Could you check a few things on this model? Use its own coordinates, in mm. A direction names the side the tool comes from. Round coordinates to 2 decimals unless told otherwise and drop trailing zeros. Order: outer loops, then holes, each group sorted by start corner. A loop starts at its lowest first (then second) coordinate and runs counter-clockwise, first axis right, second up. Notation, with made-up numbers: (22.5, 79.25) - (75.5, 79.25) arc R31 cw to (75.5, 105.25) - close; hole circle Ø6 at (-40, 71). An arc over 180 degrees is marked (long way). Use one line per item in the form item = value.
from build123d import *

# Parameters (mm, degrees)
EXTRUDE_1_DEPTH     = 1.5
SKETCH_3_R          = 2.9
EXTRUDE_2_DEPTH     = 3.829
EXTRUDE_START       = 0.5
SKETCH_4_R          = 2.9
EXTRUDE_3_DEPTH     = 0.5
SKETCH_5_R          = 2
CUT_EXTRUDE_1_DEPTH = 3
CUT_EXTRUDE_START   = -0.7
SKETCH_6_R          = 2
CUT_EXTRUDE_2_DEPTH = 0.7
SKETCH_7_R          = 1.1
CUT_EXTRUDE_3_DEPTH = 3.7
SKETCH_8_R          = 0.75
CUT_EXTRUDE_4_DEPTH = 3.7


with BuildPart() as part:
    # 草图1 → 凸台-拉伸1 (new body)
    with BuildSketch(Plane.XY):
        with BuildLine():
            Line((-2.15, 0), (-2.797439847, -4.825584994))
            ThreePointArc((-2.797439847, -4.825584994), (0, -8.49), (2.797439847, -4.825584994))
            Line((2.797439847, -4.825584994), (2.15, 0))
            ThreePointArc((2.15, 0), (0, 2.15), (-2.15, 0))
        make_face()
    extrude(amount=EXTRUDE_1_DEPTH)

    # 草图3 → 凸台-拉伸2 (add)
    with BuildSketch(Plane.XY.offset(1.5)):
        with Locations(Location((0, -5.59, 0), (0, 0, 164.716730752))):
            Circle(SKETCH_3_R)
    extrude(amount=EXTRUDE_2_DEPTH)

    # 草图4 → 凸台-拉伸3 (add)
    with BuildSketch(Plane(origin=(0, 0, 0), x_dir=(-1, 0, 0), z_dir=(0, 0, -1)).offset(EXTRUDE_START)):
        with Locations((0, -5.59)):
            Circle(SKETCH_4_R)
    extrude(amount=-EXTRUDE_3_DEPTH)

    # 草图5 → 切除-拉伸1 (cut)
    with BuildSketch(Plane.XY.offset(5.329)):
        with Locations((0, -5.59)):
            Circle(SKETCH_5_R)
    extrude(amount=-CUT_EXTRUDE_1_DEPTH, mode=Mode.SUBTRACT)

    # 草图6 → 切除-拉伸2 (cut)
    with BuildSketch(Plane(origin=(0, 0, -0.5), x_dir=(-1, 0, 0), z_dir=(0, 0, -1)).offset(CUT_EXTRUDE_START)):
        with Locations(Location((0, -5.59, 0), (0, 0, 180))):
            Circle(SKETCH_6_R)
    extrude(amount=CUT_EXTRUDE_2_DEPTH, mode=Mode.SUBTRACT)

    # 草图7 → 切除-拉伸3 (cut)
    with BuildSketch(Plane(origin=(0, 0, 0.2), x_dir=(-1, 0, 0), z_dir=(0, 0, -1))):
        with Locations((0, -5.59)):
            Circle(SKETCH_7_R)
    extrude(amount=-CUT_EXTRUDE_3_DEPTH, mode=Mode.SUBTRACT)

    # 草图8 → 切除-拉伸4 (cut)
    with BuildSketch(Plane.XY.offset(1.5)):
        Circle(SKETCH_8_R)
    extrude(amount=-CUT_EXTRUDE_4_DEPTH, mode=Mode.SUBTRACT)


solid = part.part
Item 1: For faces 5 (the face through (0.9, -4.7, 0.2)), 6 (the face through (-2.47, -2.38, 0.74)), 7 (the face through (-0.434, -7.542, 3.85)), which set-ups out of +Z, -Z, +X, -X, +Y, -Y let a thin tool reach every point of the face, with its end or its side?
Found:
face_5 = -Z
face_6 = +Z, -Z, -X, +Y
face_7 = +Z
Item 2: Imagine slicing it at A-A on y = -5.59. Please give me the cut outline in (x, z), plus the area to 3 significant figures.
Found:
outline = (-2.9, -0.5) - (-2, -0.5) - (-2, 0.2) - (-1.1, 0.2) - (-1.1, 2.33) - (-2, 2.33) - (-2, 5.33) - (-2.9, 5.33) - close; (1.1, 0.2) - (2, 0.2) - (2, -0.5) - (2.9, -0.5) - (2.9, 5.33) - (2, 5.33) - (2, 2.33) - (1.1, 2.33) - close
area = 14.3 mm2
Item 3: I need wall thicknesses on L1, parallel to Y at x = 0, z = 0.35; L2, parallel to Y at x = 0, z = -0.1; L3, parallel to Y at x = 0.3, z = 0.35. Which ranges of each line are inside material? Lowest first, please.
Found:
L1 = -8.49 to -6.69, -4.49 to -0.75, 0.75 to 2.15
L2 = -8.49 to -7.59, -3.59 to -2.69
L3 = -8.47 to -6.65, -4.53 to -0.69, 0.69 to 2.13
Item 4: Imagine slicing it at D-D on y = -3.25. Please give me the cut outline in (x, z), plus the area to 3 significant figures.
Found:
outline = (-2.59, 0) - (-1.71, 0) - (-1.71, -0.5) - (1.71, -0.5) - (1.71, 0) - (2.59, 0) - (2.59, 1.5) - (1.71, 1.5) - (1.71, 5.33) - (-1.71, 5.33) - (-1.71, 1.5) - (-2.59, 1.5) - close
area = 22.6 mm2
Item 5: If we mould it in two halves opening along Y, with no side actions, what happens to faces 1 (the face through (0.9, -6.5, 2.329)), 2 (the face through (-0.26, -7.573, -0.145)), 3 (the face through (0.05, 2.15, 0.74)), 4 (the face through (0, -1, 1.5))? For each: released by +Y, released by -Y, zero draft, split by the parting line, or undercut.
Found:
face_1 = undercut
face_2 = undercut
face_3 = released by +Y
face_4 = zero draft
Item 6: Will these pins go through, and if not, where does the flat tip stop? P1, Ø1.5, axis at x = -1.5, z = 0.5, coming from the +Y side; P2, Ø3, axis at x = 0, y = -5.59, coming from the +Z side; P3, Ø2, axis at y = -4, z = 1.5, coming from the +X side.
Found:
P1 = 2.01
P2 = 2.33
P3 = 2.84
Item 7: Imagine slicing it at B-B on x = 0. Please give me the cut outline in (y, z), plus the area to 3 significant figures.
Found:
outline = (-8.49, -0.5) - (-7.59, -0.5) - (-7.59, 0.2) - (-6.69, 0.2) - (-6.69, 2.33) - (-7.59, 2.33) - (-7.59, 5.33) - (-8.49, 5.33) - close; (-4.49, 0.2) - (-3.59, 0.2) - (-3.59, -0.5) - (-2.69, -0.5) - (-2.69, 0) - (-0.75, 0) - (-0.75, 1.5) - (-2.69, 1.5) - (-2.69, 5.33) - (-3.59, 5.33) - (-3.59, 2.33) - (-4.49, 2.33) - close; (0.75, 0) - (2.15, 0) - (2.15, 1.5) - (0.75, 1.5) - close
area = 19.3 mm2
Item 8: Imagine slicing it at C-C on z = 1.35. Please give me the cut outline in (x, y), plus the area to 3 significant figures.
Found:
outline = (-2.8, -4.83) arc R2.9 ccw (long way) to (2.8, -4.83) - (2.15, 0) arc R2.15 ccw to (-2.15, 0) - close; hole circle Ø2.2 at (0, -5.59); hole circle Ø1.5 at (0, 0)
area = 43.2 mm2
